from build123d import *

# Parameters (mm, degrees)
SKETCH1_R             = 76.2
BILLET_DEPTH          = 50.8
SKETCH3_R             = 19.05
LOX_PLATE_DEPTH       = 13.97
SKETCH5_R             = 13.97
LOX_DOME_DEPTH        = 20.32
SKETCH7_R             = 76.2
TOP_MILL_DEPTH        = 17.78
F_1_4_BOLT_HOLE_REACH = 114.708
SKETCH11_R            = 3.175
BOLT_PATTERN_COUNT    = 8
SKETCH12_R            = 57.15
KEROSENE_PLATE_DEPTH  = 10.16
KEROSENE_INLET_REACH  = 121.137
SKETCH13_R            = 4.7625
MANIFOLD_HOLE_REACH   = 121.137
SKETCH14_R            = 3.175
SKETCH15_R            = 10.16
SKETCH15_R_2          = 7.62
MANIFOLD_SEAL_DEPTH   = 12.192


with BuildPart() as part:
    # Sketch1 → Billet (new body)
    with BuildSketch(Plane(origin=(0, 0, 0), x_dir=(1, 0, 0), z_dir=(0, 1, 0))):
        with Locations(Location((0, 0, 0), (0, 0, 270))):
            Circle(SKETCH1_R)
    extrude(amount=-BILLET_DEPTH)

    # Sketch3 → Lox Plate (cut)
    with BuildSketch(Plane(origin=(0, -50.8, 0), x_dir=(1, 0, 0), z_dir=(0, 1, 0))):
        with Locations(Location((0, 0, 0), (0, 0, 270))):
            Circle(SKETCH3_R)
    extrude(amount=LOX_PLATE_DEPTH, mode=Mode.SUBTRACT)

    # Sketch5 → Lox Dome (cut)
    with BuildSketch(Plane(origin=(0, -50.8, 0), x_dir=(1, 0, 0), z_dir=(0, 1, 0))):
        with Locations(Location((0, 0, 0), (0, 0, 270))):
            Circle(SKETCH5_R)
    extrude(amount=LOX_DOME_DEPTH, mode=Mode.SUBTRACT)

    # Sketch7 → Top Mill (cut)
    with BuildSketch(Plane(origin=(0, 0, 0), x_dir=(1, 0, 0), z_dir=(0, 1, 0))):
        with Locations(Location((0, 0, 0), (0, 0, 270))):
            Circle(SKETCH7_R)
    extrude(amount=-TOP_MILL_DEPTH, mode=Mode.SUBTRACT)

    # Sketch11 → 1_4_ Bolt Hole (cut, up to next)
    with BuildSketch(Plane(origin=(0, -50.8, 0), x_dir=(1, 0, 0), z_dir=(0, 1, 0)), mode=Mode.PRIVATE) as f_1_4_bolt_hole_sk1:
        with Locations(Location((0, 68.58, 0), (0, 0, 270))):
            Circle(SKETCH11_R)
    f_1_4_bolt_hole_tool1 = extrude(f_1_4_bolt_hole_sk1.sketch, amount=F_1_4_BOLT_HOLE_REACH, mode=Mode.PRIVATE) & part.part
    f_1_4_bolt_hole = f_1_4_bolt_hole_tool1.solids().sort_by_distance((0, -50.8, -68.58))[0]
    add(f_1_4_bolt_hole, mode=Mode.SUBTRACT)

    # Bolt Pattern: 1_4_ Bolt Hole ×8 about axis
    bolt_pattern_axis = Axis((0, 0, 0), (0, 1, 0))
    for i in range(1, BOLT_PATTERN_COUNT):
        add(f_1_4_bolt_hole.rotate(bolt_pattern_axis, i * 360 / BOLT_PATTERN_COUNT), mode=Mode.SUBTRACT)

    # Sketch12 → Kerosene Plate (cut)
    with BuildSketch(Plane(origin=(0, -50.8, 0), x_dir=(1, 0, 0), z_dir=(0, 1, 0))):
        with Locations(Location((0, 0, 0), (0, 0, 270))):
            Circle(SKETCH12_R)
    extrude(amount=KEROSENE_PLATE_DEPTH, mode=Mode.SUBTRACT)

    # Sketch13 → Kerosene Inlet (cut, up to next)
    with BuildSketch(Plane(origin=(0, 0, 0), x_dir=(1, 0, 0), z_dir=(0, 1, 0)), mode=Mode.PRIVATE) as kerosene_inlet_sk1:
        with Locations(Location((-31.75, 0, 0), (0, 0, 270))):
            Circle(SKETCH13_R)
    kerosene_inlet_tool1 = extrude(kerosene_inlet_sk1.sketch, amount=-KEROSENE_INLET_REACH, mode=Mode.PRIVATE) & part.part
    # Sketch13 → Kerosene Inlet (cut, up to next)
    with BuildSketch(Plane(origin=(0, 0, 0), x_dir=(1, 0, 0), z_dir=(0, 1, 0)), mode=Mode.PRIVATE) as kerosene_inlet_sk2:
        with Locations(Location((31.75, 0, 0), (0, 0, 270))):
            Circle(SKETCH13_R)
    kerosene_inlet_tool2 = extrude(kerosene_inlet_sk2.sketch, amount=-KEROSENE_INLET_REACH, mode=Mode.PRIVATE) & part.part
    add(kerosene_inlet_tool1.solids().sort_by_distance((-31.75, 0, 0))[0], mode=Mode.SUBTRACT)
    add(kerosene_inlet_tool2.solids().sort_by_distance((31.75, 0, 0))[0], mode=Mode.SUBTRACT)

    # Sketch14 → Manifold hole (cut, up to next)
    with BuildSketch(Plane(origin=(0, 0, 0), x_dir=(1, 0, 0), z_dir=(0, 1, 0)), mode=Mode.PRIVATE) as manifold_hole_sk1:
        with Locations(Location((0, 33.02, 0), (0, 0, 270))):
            Circle(SKETCH14_R)
    manifold_hole_tool1 = extrude(manifold_hole_sk1.sketch, amount=-MANIFOLD_HOLE_REACH, mode=Mode.PRIVATE) & part.part
    add(manifold_hole_tool1.solids().sort_by_distance((0, 0, -33.02))[0], mode=Mode.SUBTRACT)

    # Sketch15 → Manifold seal (cut)
    with BuildSketch(Plane(origin=(0, -50.8, 0), x_dir=(1, 0, 0), z_dir=(0, 1, 0))):
        with Locations(Location((0, 33.02, 0), (0, 0, 90))):
            Circle(SKETCH15_R)
        with Locations(Location((0, 33.02, 0), (0, 0, 90))):
            Circle(SKETCH15_R_2, mode=Mode.SUBTRACT)
    extrude(amount=MANIFOLD_SEAL_DEPTH, mode=Mode.SUBTRACT)

    # Sketch21 → 1_2 NPT Tapped Hole3 (revolve, cut)
    with BuildSketch(Plane(origin=(0, -17.78, 0), x_dir=(0, 0, 1), z_dir=(1, 0, 0))):
        Polygon((0, 0), (0, 33.02), (8.9281, 33.02), (8.9281, 13.462), (9.479726792, 13.462), (9.8827971, 0), align=None)
    revolve(axis=Axis((0, -11.43, 0), (0, -1, 0)), mode=Mode.SUBTRACT)


solid = part.part
Geometry: final body of the model. Coordinates: model frame, mm. A direction names the side the tool comes from. Give positions to 0.01 mm unless a question says otherwise; leave off trailing zeros. Write each loop counter-clockwise with the first axis right and the second up, starting at its lowest first coordinate (ties: lowest second). Pieces come first, ordered by that corner, then holes. Notation, with made-up numbers: M 66.5,-13.5 L 104.5,-13.5 A16 ccw 104.5,4.5 Z; hole C 45,49 d5. An arc over 180 degrees is marked long. Answer in a Markdown table with one row per item. Add a question column.
(1) Section B-B on x = -68.58. Return loops of the section in (y, z) (3 decimals), and give its area (3 significant figures).
(2) Reachability of faces 4 (the cylindrical face through (71.75, -34.52, 0.14)), 5 (the flat face through (-8, -38.608, -34)) from +Z, -Z, +X, -X, +Y, -Y: full face, straight path, thin tool, end or side. Return the list, or none.
(3) Section A-A on z = 68.58. Return loops of the section in (x, y) (3 decimals).
(4) Mould query, pull axis X, two halves, no side actions, for faces 1 (the cylindrical face through (13.85, -33.7, -1.82)), 2 (the cylindrical face through (-46.367, -34.059, -60.47)), 3 (the flat face through (51, -50.8, -29)). Classes: +X half, -X half, draft (parallel to the pull), parting line (faces both ways), or undercut.
(5) Ray query, line 1 (X direction, y = -41.5, z = 50.5); line 2 (X direction, y = -37, z = 56); line 3 (Y direction, x = -8, z = -22.5). Return the intervals inside material, ascending.
(6) First-contact query: pin 1 (1.5 mm diameter, centred on x = -9.5, z = 48, fed in from -Y); pin 2 (5 mm diameter, centred on x = 0, z = -33.02, fed in from +Y); pin 3 (8 mm diameter, centred on y = -23, z = -22, fed in from +X); pin 4 (6 mm diameter, centred on y = -44.5, z = 9, fed in from -X). Flat tips, straight axial feed; report the tip coordinate or a pass-through.
(7) Section C-C on y = -22. State how many separate pieces and enclosed holes the cut face has, and give its area (3 significant figures).
(8) Section D-D on x = 38.5. Return loops of the section in (y, z).
Result set:
| question | item | result |
|---|---|---|
| 1 | outline | M -50.8,-33.215 L -17.78,-33.215 L -17.78,-3.175 L -50.8,-3.175 Z; M -50.8,3.175 L -17.78,3.175 L -17.78,33.215 L -50.8,33.215 Z |
| 1 | area | 1,980 mm^2 |
| 2 | face 4 | +Y, -Y |
| 2 | face 5 | -Y |
| 3 | outline | M -33.215,-50.8 L -3.175,-50.8 L -3.175,-17.78 L -33.215,-17.78 Z; M 3.175,-50.8 L 33.215,-50.8 L 33.215,-17.78 L 3.175,-17.78 Z |
| 4 | face 1 | undercut |
| 4 | face 2 | parting line |
| 4 | face 3 | draft |
| 5 | line 1 | x = -57.06 to -50.95, -46.03 to -26.76, 26.76 to 46.03, 50.95 to 57.06 |
| 5 | line 2 | x = -51.68 to 51.68 |
| 5 | line 3 | y = -40.64 to -17.78 |
| 6 | pin 1 | stops at y = -40.64 |
| 6 | pin 2 | passes through |
| 6 | pin 3 | stops at x = 74.04 |
| 6 | pin 4 | stops at x = -75.96 |
| 7 | separate pieces | 1 |
| 7 | enclosed holes | 12 |
| 7 | area | 17,500 mm^2 |
| 8 | outline | M -50.8,-65.76 L -17.78,-65.76 L -17.78,65.76 L -50.8,65.76 L -50.8,42.24 L -40.64,42.24 L -40.64,-42.24 L -50.8,-42.24 Z |
